Here's the drawing with two shaded views (mm, measured from the low corner). I have some questions. Round coordinates to 2 decimals unless told otherwise and drop trailing zeros. Loops run counter-clockwise (first coordinate to the right, second up) from the corner with the lowest first, then second, coordinate; pieces in that order, holes last.
(1) If I drill on line 1 along Z through (x, y) = (23.75, 15.25); line 2 along Y through (x, z) = (13.25, 230.5); line 3 along X through (y, z) = (12.25, 132), over which ranges is the centre line in solid material (lowest first)?
(2) I want a section at B-B on z = 229. Write out the boundary of the cut face in (x, y).
(3) Will these pins go through, and if not, where does the flat tip stop? pin 1 Ø1 at (y, z) = (16, 74) entering from +X; pin 2 Ø12 at (x, z) = (18, 141) entering from -Y; pin 3 Ø1.5 at (x, z) = (9, 58) entering from -Y.
(4) I want a section at A-A on x = 13. Write out the boundary of the cut face in (y, z).
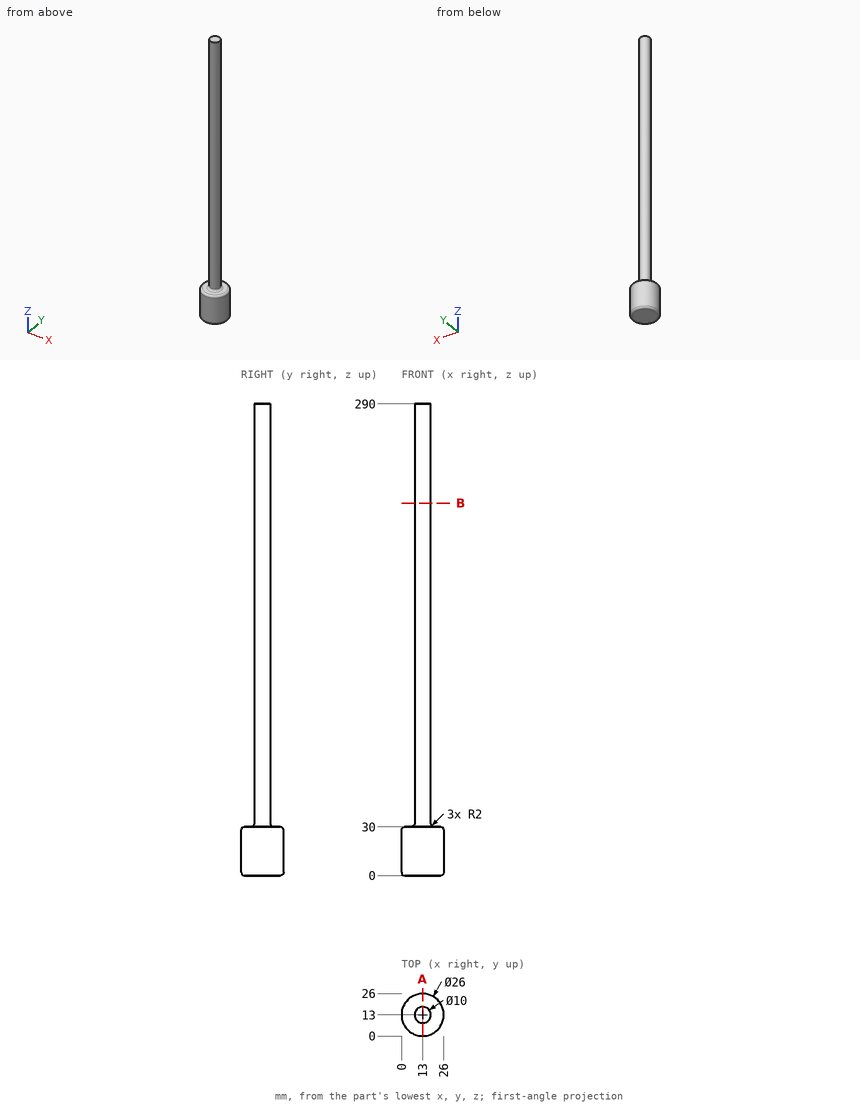
Filled sheet:
1. line 1: z = 0 to 30
1. line 2: y = 8.01 to 17.99
1. line 3: x = 8.06 to 17.94
2. outline: circle Ø10 at (13, 13)
3. pin 1: stops at x = 17.33
3. pin 2: stops at y = 8
3. pin 3: stops at y = 9.2
4. outline: (0, 2) arc R2 ccw to (2, 0) - (24, 0) arc R2 ccw to (26, 2) - (26, 28) arc R2 ccw to (24, 30) - (20, 30) arc R2 cw to (18, 32) - (18, 290) - (8, 290) - (8, 32) arc R2 cw to (6, 30) - (2, 30) arc R2 ccw to (0, 28) - close
